```python
from build123d import *
from build123d.topology import SkipClean

# Parameters (mm, degrees)
SKETCH10_R              = 10
BOSS_EXTRUDE1_DEPTH     = 5
CUT_EXTRUDE3_DEPTH      = 45
CUT_EXTRUDE3_DEPTH_BACK = 20


with BuildPart() as part:
    # Sketch1 → Revolve1 (revolve)
    with BuildSketch(Plane.XY):
        with BuildLine():
            Line((20.9, 0), (23.871591838, 0))
            Line((23.871591838, 0), (23.871591838, 4))
            Line((23.871591838, 4), (22.9, 4.236662843))
            Line((22.9, 4.236662843), (22.9, 11.404308102))
            ThreePointArc((22.9, 11.404308102), (23.83692213, 15.63049072), (26.472123903, 19.064752533))
            Line((26.472123903, 19.064752533), (26.988320528, 19.497892931))
            ThreePointArc((26.988320528, 19.497892931), (29.623522302, 22.932154745), (30.560444431, 27.158337362))
            Line((30.560444431, 27.158337362), (30.560444431, 50))
            ThreePointArc((30.560444431, 50), (29.388871556, 52.828427125), (26.560444431, 54))
            Line((26.560444431, 54), (2.764914955, 54))
            Line((2.764914955, 54), (2.764914955, 15))
            Line((2.764914955, 15), (19.9, 15))
            ThreePointArc((19.9, 15), (20.607106781, 14.707106781), (20.9, 14))
            Line((20.9, 14), (20.9, 0))
        make_face()
    revolve(axis=Axis((2.764914955, 7.821821657, 0), (0, 1, 0)))

    # Sketch10 → Boss-Extrude1 (add)
    with SkipClean():  # the faces are left unmerged after this step: merging them gives an invalid solid
        with BuildSketch(Plane.XY.offset(27.795529476)):
            with Locations((3.346345887, 38.658337362)):
                Circle(SKETCH10_R)
        extrude(amount=-BOSS_EXTRUDE1_DEPTH)

    # Sketch11 → Cut-Extrude3 (cut, two sides: drawn at the far end of the back side and taken through both)
    with SkipClean():  # the faces are left unmerged after this step: merging them gives an invalid solid
        with BuildSketch(Plane(origin=(0, 17, 0), x_dir=(1, 0, 0), z_dir=(0, 1, 0)).offset(-CUT_EXTRUDE3_DEPTH_BACK)):
            with BuildLine():
                Line((-14.735085045, 0), (20.264914955, 0))
                ThreePointArc((20.264914955, 0), (2.764914955, 17.5), (-14.735085045, 0))
            make_face()
        extrude(amount=CUT_EXTRUDE3_DEPTH + CUT_EXTRUDE3_DEPTH_BACK, mode=Mode.SUBTRACT)


solid = part.part
```
Read the model definition and answer for the solid it produces. Units are mm, in the model's axes. A direction names the side the tool comes from. Round coordinates to 2 decimals unless told otherwise and drop trailing zeros. Write each loop counter-clockwise with the first axis right and the second up, starting at its lowest first coordinate (ties: lowest second). Pieces come first, ordered by that corner, then holes. Notation, with made-up numbers: (36.5, 65) - (51.5, 65) arc R17 ccw to (51.5, 76) - close; hole circle Ø7 at (-29, 16). An arc over 180 degrees is marked (long way). One line per item, written item: value.
Q1. For a pull along X with two mould halves and no side action, classify faces 1 (the flat face through (-7, 0, -16)), 2 (the flat face through (3, 34, 0)), 3 (the cylindrical face through (-13.214, 7.871, 12.252)), 4 (the flat face through (3, 15, 7)) as pulls with the +X half, pulls with the -X half, needs draft (parallel to the pull), parting line crosses it, or undercut.
The answers:
face 1: needs draft
face 2: undercut
face 3: parting line crosses it
face 4: undercut
Q2. Find section A-A (y = 35). Determine the outline of the cut face in (x, z), and give its area (3 significant figures).
The answers:
outline: (-5.96, 26.39) arc R27.8 ccw (long way) to (12.65, 25.98) - (12.65, 27.8) - (-5.96, 27.8) - close; hole (-14.74, 0) arc R17.5 ccw to (20.26, 0) - close
area: 1,960 mm2
Q3. Straight lines are drawn through the part: line 1 (X direction, y = 10, z = 0); line 2 (X direction, y = 3, z = 0); line 3 (Z direction, x = 3.5, y = 28.5). For each, find the intervals that lie inside material, in ascending order. Write a range as from..to.
The answers:
line 1: x = -17.37..-15.37, 20.9..22.9
line 2: x = -18.34..-15.37, 20.9..23.87
line 3: z = -27.79..-17.48, 0..27.79
Q4. Each of these flat-tipped pins is pushed along its axis until it touches: P1, Ø1, axis at y = 35.5, z = -22, coming from the -X side; P2, Ø5, axis at x = -8, y = 6.5, coming from the -Z side; P3, Ø3, axis at x = -13.5, y = 18.5, coming from the -Z side. Where does it stop, or does it pass through?
The answers:
P1: stops at x = -14.85
P2: stops at z = -18.36
P3: stops at z = -19.05
Q5. Which of the six approach directions +Z, -Z, +X, -X, +Y, -Y give full straight-line access (tool end or side, diameter ignored) to faces 5 (the cylindrical face through (3.15, 34.192, -17.496)), 6 (the flat face through (2, 54, 5)), 7 (the cylindrical face through (-1.811, 2.028, 20.605))?
The answers:
face 5: +Y, -Y
face 6: +Z, -Z, +X, -X, +Y
face 7: -Y
Q6. Find section B-B (y = 22.5). Determine the outline of the cut face in (x, z), and give its area (3 significant figures).
The answers:
outline: circle Ø53.29 at (2.76, 0); hole (-14.74, 0) arc R17.5 ccw to (20.26, 0) - close
area: 1,750 mm2
